from build123d import *

# Parameters (mm, degrees)
F0_R          = 2.125
F0_R_2        = 4.25
F0_R_3        = 3.25
F1_DEPTH      = 5
F2_W          = 25
F2_H          = 5
F3_DEPTH      = 25
F4_R          = 8.25
F4_R_2        = 4.25
F4_R_3        = 7.25
F4_R_4        = 3.25
F5_DEPTH      = 10
F6_R          = 2.125
F7_DEPTH      = 5.001
F8_W          = 5
F8_H          = 13.6379074032
F8_W_2        = 4
F8_H_2        = 16.0665388563
F9_DEPTH      = 10
F10_T1_DEPTH  = 5
F10_T3_DEPTH  = 4
F10_T8_DEPTH  = 17.8584149398
F10_T13_DEPTH = 16.8584149398
F10_T18_DEPTH = 26.4963223431
F10_S19_R     = 8.25
F10_T20_DEPTH = 15
F10_T25_DEPTH = 26.4963223431
F10_S26_R     = 8.25
F10_T27_DEPTH = 15
F10_T32_DEPTH = 27.1526880508
F10_S34_R     = 7.25
F10_T35_DEPTH = 16


# Not quite as in the source:
# - a fillet or chamfer that OpenCascade refuses, or shapes differently, is made with other operations: its cross-section is extruded or revolved along the edge and cut away or added


with BuildPart() as f1:
    # F0 (on Top) → F1 (new body)
    with BuildSketch(Plane.XY):
        with BuildLine():
            Line((12.5, 26.5), (0, 26.5))
            Line((0, 26.5), (-12.5, 26.5))
            Line((-12.5, 26.5), (-12.5, 6.5622023742))
            ThreePointArc((-12.5, 6.5622023742), (-15.3166703137, -2.6385915194), (-7.5, -8.25))
            Line((-7.5, -8.25), (-7.5, -13.6))
            ThreePointArc((-7.5, -13.6), (-5.3033008589, -18.9033008589), (0, -21.1))
            ThreePointArc((0, -21.1), (5.3033008589, -18.9033008589), (7.5, -13.6))
            Line((7.5, -13.6), (7.5, -7.0478720193))
            Line((7.5, -7.0478720193), (12.5, -7.0478720193))
            ThreePointArc((12.5, -7.0478720193), (18.05, 0), (12.5, 7.0478720193))
            Line((12.5, 7.0478720193), (12.5, 26.5))
        make_face()
        with Locations((0, -13.6)):
            Circle(F0_R, mode=Mode.SUBTRACT)
        with Locations((-7.5, 0)):
            Circle(F0_R_2, mode=Mode.SUBTRACT)
        with Locations((10.8, 0)):
            Circle(F0_R_3, mode=Mode.SUBTRACT)
        with Locations((0, 16.5)):
            Circle(F0_R, mode=Mode.SUBTRACT)
    extrude(amount=F1_DEPTH)

    # F2 (on face) → F3 (join)
    with BuildSketch(Plane.XY.offset(5)):
        with Locations((0, 24)):
            Rectangle(F2_W, F2_H)
    extrude(amount=F3_DEPTH)

    # F4 (on face) → F5 (join)
    with BuildSketch(Plane.XY.offset(5)):
        with Locations((-7.5, 0)):
            Circle(F4_R)
        with Locations((-7.5, 0)):
            Circle(F4_R_2, mode=Mode.SUBTRACT)
        with Locations((10.8, 0)):
            Circle(F4_R_3)
        with Locations((10.8, 0)):
            Circle(F4_R_4, mode=Mode.SUBTRACT)
    extrude(amount=F5_DEPTH)

    # F6 (on face) → F7 (cut, through all)
    with BuildSketch(Plane.XZ.offset(-21.5)):
        with Locations((0, 22.5)):
            Circle(F6_R)
    extrude(amount=-F7_DEPTH, mode=Mode.SUBTRACT)

    # F8 (on face) → F9 (join)
    with BuildSketch(Plane.XY.offset(5)):
        with Locations((-7.5, 14.6810462984)):
            Rectangle(F8_W, F8_H)
        with Locations((8, 13.4667305718)):
            Rectangle(F8_W_2, F8_H_2)
    extrude(amount=F9_DEPTH)

    # F10: chamfer of 5 on 4 edges, made by hand

    # F10_s2 → F10_t1 (join)
    with BuildSketch(Plane.YZ.offset(-10)):
        Polygon((16.5, 15), (21.5, 20), (21.5, 15), align=None)
    extrude(amount=F10_T1_DEPTH)

    # F10_s4 → F10_t3 (join)
    with BuildSketch(Plane.YZ.offset(6)):
        Polygon((16.5, 15), (21.5, 20), (21.5, 15), align=None)
    extrude(amount=F10_T3_DEPTH)


with BuildPart() as f10_tool6:
    # F10_s7 → F10_t8 (new body)
    with BuildSketch(Plane.YZ.offset(7.8584149398)):
        Polygon((16.5, 15), (21.5, 20), (21.5, 15), align=None)
    extrude(amount=-F10_T8_DEPTH)

    split(bisect_by=Plane.YZ.offset(6), keep=Keep.TOP)


with BuildPart() as f1_1:
    add(f1.part)

    # F10_t5: union F10_tool6
    add(f10_tool6.part)


with BuildPart() as f10_tool11:
    # F10_s12 → F10_t13 (new body)
    with BuildSketch(Plane.YZ.offset(10)):
        Polygon((16.5, 15), (21.5, 20), (21.5, 15), align=None)
    extrude(amount=-F10_T13_DEPTH)

    split(bisect_by=Plane.YZ.offset(-5), keep=Keep.BOTTOM)


with BuildPart() as f1_2:
    add(f1_1.part)

    # F10_t10: union F10_tool11
    add(f10_tool11.part)


with BuildPart() as f10_tool16:
    # F10_s17 → F10_t18 (new body)
    with BuildSketch(Plane.XZ.offset(-21.5)):
        Polygon((-10, 10), (-15, 5), (-10, 5), align=None)
    extrude(amount=F10_T18_DEPTH)

    # F10_s19 → F10_t20 (cut, symmetric)
    with BuildSketch(Plane.XY.offset(7.5)):
        with Locations((-7.5, 0)):
            Circle(F10_S19_R)
    extrude(amount=F10_T20_DEPTH, both=True, mode=Mode.SUBTRACT)

    split(bisect_by=Plane.YZ.offset(-12.5), keep=Keep.TOP)


with BuildPart() as f1_3:
    add(f1_2.part)

    # F10_t15: union F10_tool16
    add(f10_tool16.part)


with BuildPart() as f10_tool23:
    # F10_s24 → F10_t25 (new body)
    with BuildSketch(Plane.XZ.offset(-21.5)):
        Polygon((-10, 10), (-15, 5), (-10, 5), align=None)
    extrude(amount=F10_T25_DEPTH)

    # F10_s26 → F10_t27 (intersect, symmetric)
    with BuildSketch(Plane.XY.offset(7.5)):
        with Locations((-7.5, 0)):
            Circle(F10_S26_R)
    extrude(amount=F10_T27_DEPTH, both=True, mode=Mode.INTERSECT)

    split(bisect_by=Plane.YZ.offset(-12.5), keep=Keep.BOTTOM)


with BuildPart() as f1_4:
    add(f1_3.part)

    # F10_t22: union F10_tool23
    add(f10_tool23.part)


with BuildPart() as f10_tool30:
    # F10_s31 → F10_t32 (new body)
    with BuildSketch(Plane.XZ.offset(5.6526880508)):
        Polygon((10, 10), (15, 5), (10, 5), align=None)
    extrude(amount=-F10_T32_DEPTH)

    split(bisect_by=Plane.YZ.offset(12.5), keep=Keep.BOTTOM)

    # F10_s34 → F10_t35 (cut, symmetric)
    with BuildSketch(Plane.XY.offset(7.5)):
        with Locations((10.8, 0)):
            Circle(F10_S34_R)
    extrude(amount=F10_T35_DEPTH, both=True, mode=Mode.SUBTRACT)


with BuildPart() as f1_5:
    add(f1_4.part)

    # F10_t29: union F10_tool30
    add(f10_tool30.part)


solid = f1_5.part
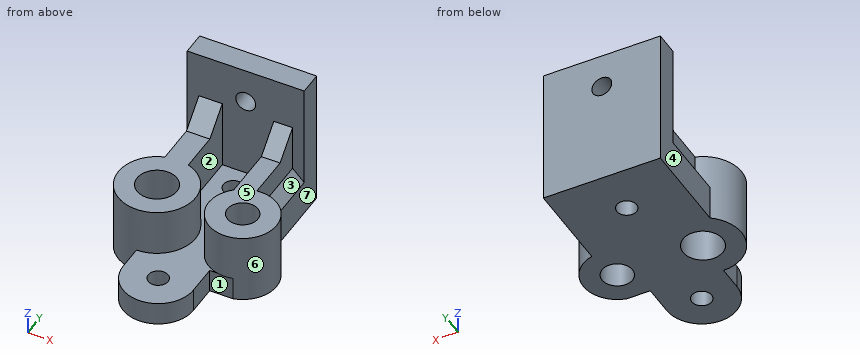
Geometry check sheet. Reference: the model listing, model coordinates, mm. Face numbers are marked on the shaded views. A direction names the side the tool comes from. Give positions to 0.01 mm unless a question says otherwise; leave off trailing zeros. Loops run counter-clockwise (first coordinate to the right, second up) from the corner with the lowest first, then second, coordinate; pieces in that order, holes last. Notation, with made-up numbers: M -38,13.25 L 15,13.25 A21 ccw 15,46.25 Z; hole C 30.25,57.5 d7. An arc over 180 degrees is marked long. Answer as a JSON object with one key per item and string values. Group by question number.
Item 1: Mould release check, pull along X, two halves, no side actions. Record for the marked faces 1, 2 and 3: pulls with the +X half, pulls with the -X half, needs draft (parallel to the pull), parting line crosses it, or undercut.
Item 2: Sectioned sample at D-D on x = 0. Record the boundary of the cut face in (y, z) (3 decimals).
Item 3: Gauge pin test, flat ends, axial feed: pin 1 (10 mm diameter, centred on x = -10, z = 14.5, fed in from -Y); pin 2 (1.5 mm diameter, centred on y = -10.5, z = 2, fed in from +X); pin 3 (8 mm diameter, centred on y = 12.5, z = 13, fed in from -X); pin 4 (3.5 mm diameter, centred on x = 0, y = 16.5, fed in from +Z). Record the tip position at first contact, or that the pin passes through.
Item 4: Access from +Z, -Z, +X, -X, +Y, -Y to the whole of each face (thin tool, end or side, straight path). Record for the marked faces 4, 5, 6 and 7.
Item 5: Sectioned sample at A-A on y = 0. Record the boundary of the cut face in (x, z).
Item 6: Material ranges on L1, parallel to Y at x = 0, z = 4 (3 decimals); L2, parallel to Z at x = 0, y = 23.85 (3 decimals); L3, parallel to Y at x = -7.5, z = 8.75, recorded low to high.
Item 7: Sectioned sample at C-C on z = 16. Record the boundary of the cut face in (x, y).
Item 8: Sectioned sample at B-B on x = 10.8. Record the boundary of the cut face in (y, z).
Findings below:
{
 "1": {"face 1": "needs draft", "face 2": "undercut", "face 3": "pulls with the +X half"},
 "2": {"outline": "M -21.1,0 L -15.725,0 L -15.725,5 L -21.1,5 Z; M -11.475,0 L 14.375,0 L 14.375,5 L 3.437,5 L 3.437,15 L -3.437,15 L -3.437,5 L -11.475,5 Z; M 18.625,0 L 26.5,0 L 26.5,20.375 L 21.5,20.375 L 21.5,5 L 18.625,5 Z; M 21.5,24.625 L 26.5,24.625 L 26.5,30 L 21.5,30 Z"},
 "3": {"pin 1": "y = -8.25", "pin 2": "x = 7.5", "pin 3": "x = -11", "pin 4": "through"},
 "4": {"face 4": "+Z, -Z, -X, +Y", "face 5": "+Z, +X, -X, -Y", "face 6": "+Z", "face 7": "+Z, -Z, +X, +Y"},
 "5": {"outline": "M -15.75,0 L -11.75,0 L -11.75,15 L -15.75,15 Z; M -3.25,0 L 7.55,0 L 7.55,15 L 3.55,15 L 3.55,5 L 0.75,5 L 0.75,15 L -3.25,15 Z; M 14.05,0 L 18.05,0 L 18.05,15 L 14.05,15 Z"},
 "6": {"L1": "-21.1 to -15.725, -11.475 to 14.375, 18.625 to 26.5", "L2": "0 to 20.375, 24.625 to 30", "L3": "-8.25 to -4.25, 4.25 to 26.5"},
 "7": {"outline": "M -12.5,21.5 L -10,21.5 L -10,17.5 L -5,17.5 L -5,21.5 L 6,21.5 L 6,17.5 L 10,17.5 L 10,21.5 L 12.5,21.5 L 12.5,26.5 L -12.5,26.5 Z"},
 "8": {"outline": "M -7.25,5 L -7.05,5 L -7.05,0 L -3.25,0 L -3.25,15 L -7.25,15 Z; M 3.25,0 L 26.5,0 L 26.5,30 L 21.5,30 L 21.5,9.2 L 7.25,9.2 L 7.25,15 L 3.25,15 Z"}
}
